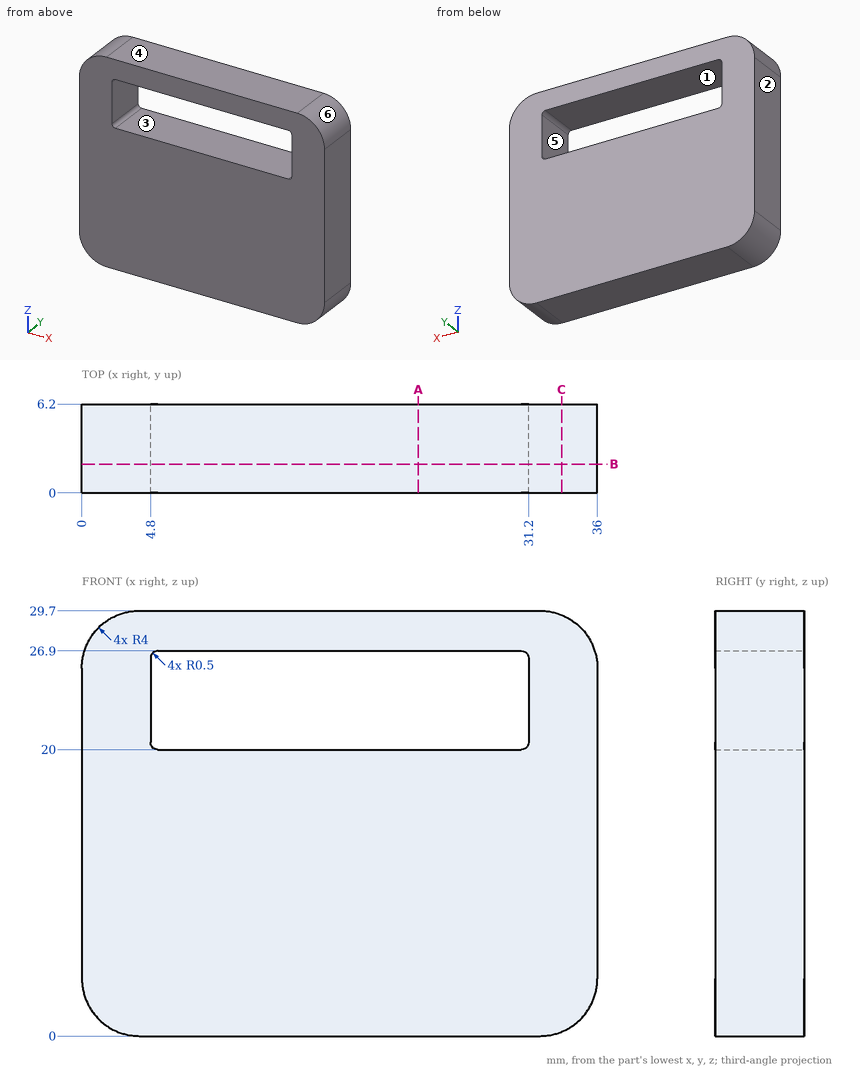
Verification items for this drawing (mm, ordinates from the low corner). A direction names the side the tool comes from. Coordinates: 2 decimals unless noted, no trailing zeros. Loops run counter-clockwise (first coordinate to the right, second up) from the corner with the lowest first, then second, coordinate; pieces in that order, holes last. Notation, with made-up numbers: (87, 39.5) - (100, 39.5) arc R24 cw to (100, 49.5) - close; hole circle Ø5 at (51, -26). An arc over 180 degrees is marked (long way). Answer as a JSON object with one key per item and string values.
(1) Cross-section at B-B, the plane y = 2. Record the boundary of the cut face in (x, z), then the cut area to 3 significant figures.
Response:
{"outline": "(0, 4) arc R4 ccw to (4, 0) - (32, 0) arc R4 ccw to (36, 4) - (36, 25.7) arc R4 ccw to (32, 29.7) - (4, 29.7) arc R4 ccw to (0, 25.7) - close; hole (4.8, 20.5) arc R0.5 ccw to (5.3, 20) - (30.7, 20) arc R0.5 ccw to (31.2, 20.5) - (31.2, 26.4) arc R0.5 ccw to (30.7, 26.9) - (5.3, 26.9) arc R0.5 ccw to (4.8, 26.4) - close", "area": "874 mm²"}
(2) Cross-section at A-A, the plane x = 23.5. Record the boundary of the cut face in (y, z), then the cut area to 3 significant figures.
Response:
{"outline": "(0, 0) - (6.2, 0) - (6.2, 20) - (0, 20) - close; (0, 26.9) - (6.2, 26.9) - (6.2, 29.7) - (0, 29.7) - close", "area": "141 mm²"}
(3) Scan lines: line 1 along Z through (x, y) = (10, 2.5); line 2 along X through (y, z) = (3.25, 22); line 3 along Z through (x, y) = (34, 1.5). Record each from-to range of solid material in increasing order.
Response:
{"line 1": "z = 0 to 20, 26.9 to 29.7", "line 2": "x = 0 to 4.8, 31.2 to 36", "line 3": "z = 0.54 to 29.16"}
(4) Access from +Z, -Z, +X, -X, +Y, -Y to the whole of each face (thin tool, end or side, straight path). Record for the marked faces 5 and 6.
Response:
{"face 5": "+Y, -Y", "face 6": "+Z, +X, +Y, -Y"}
(5) Mould release check, pull along X, two halves, no side actions. Record for the marked faces 1, 2, 3 and 4: pulls with the +X half, pulls with the -X half, needs draft (parallel to the pull), parting line crosses it, or undercut.
Response:
{"face 1": "undercut", "face 2": "pulls with the -X half", "face 3": "undercut", "face 4": "needs draft"}
(6) Cross-section at C-C, the plane x = 33.5. Record the boundary of the cut face in (y, z), then the cut area to 3 significant figures.
Response:
{"outline": "(0, 0.29) - (6.2, 0.29) - (6.2, 29.41) - (0, 29.41) - close", "area": "181 mm²"}
(7) Go/stop test with a flat-tipped pin: pin 1 Ø3 at (x, y) = (17.5, 3.5) entering from -Z. Record where the tip stops, or that it passes through.
Response:
{"pin 1": "stops at z = 0"}
